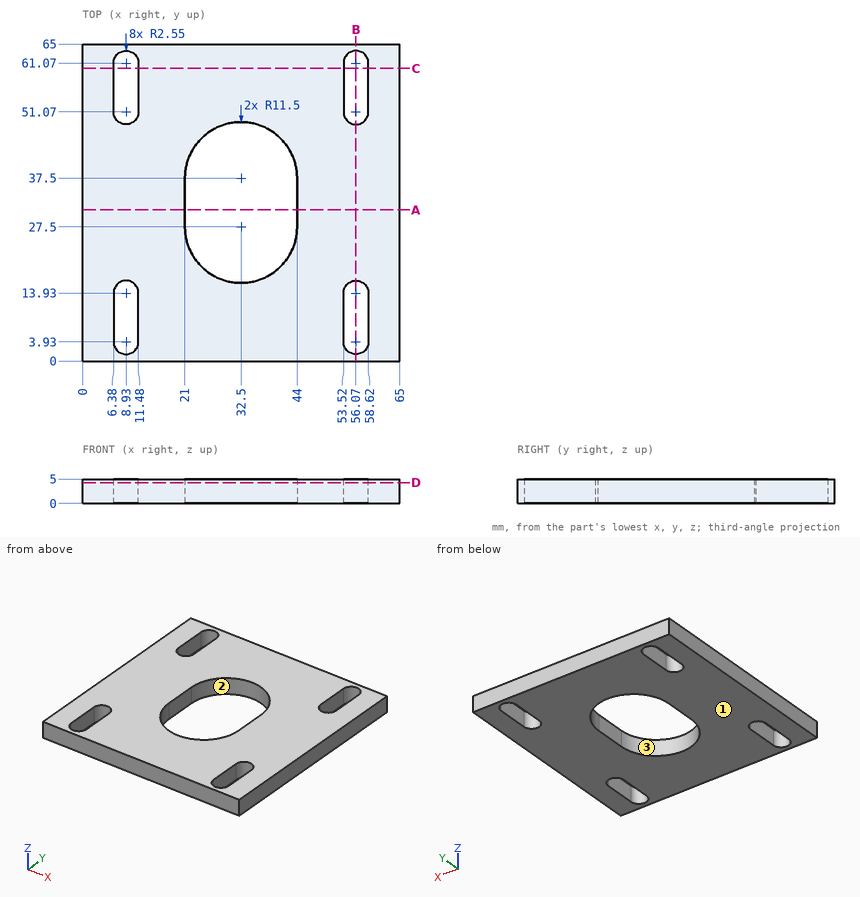
Here's the drawing with two shaded views (mm, measured from the low corner). I have some questions. Coordinates: 2 decimals unless noted, no trailing zeros. Order: outer loops, then holes, each group sorted by start corner. A loop starts at its lowest first (then second) coordinate and runs counter-clockwise, first axis right, second up. Notation, with made-up numbers: (84, 85) - (116, 85) arc R23 cw to (116, 107) - close; hole circle Ø3 at (61.5, -31). An arc over 180 degrees is marked (long way). Answer in a Markdown table with one row per item.
1. Suppose I cut it at D-D (z = 4.25). Please give me the cut outline in (x, y), and give its area (3 significant figures).
Reply:
| item | result |
|---|---|
| outline | (0, 0) - (65, 0) - (65, 65) - (0, 65) - close; hole (6.38, 3.93) arc R2.55 ccw to (11.48, 3.93) - (11.48, 13.93) arc R2.55 ccw to (6.38, 13.93) - close; hole (6.38, 51.07) arc R2.55 ccw to (11.48, 51.07) - (11.48, 61.07) arc R2.55 ccw to (6.38, 61.07) - close; hole (21, 27.5) arc R11.5 ccw to (44, 27.5) - (44, 37.5) arc R11.5 ccw to (21, 37.5) - close; hole (53.52, 3.93) arc R2.55 ccw to (58.62, 3.93) - (58.62, 13.93) arc R2.55 ccw to (53.52, 13.93) - close; hole (53.52, 51.07) arc R2.55 ccw to (58.62, 51.07) - (58.62, 61.07) arc R2.55 ccw to (53.52, 61.07) - close |
| area | 3,290 mm^2 |
2. Suppose I cut it at C-C (y = 60). Please give me the cut outline in (x, z), and give its area (3 significant figures).
Reply:
| item | result |
|---|---|
| outline | (0, 0) - (6.38, 0) - (6.38, 5) - (0, 5) - close; (11.48, 0) - (53.52, 0) - (53.52, 5) - (11.48, 5) - close; (58.62, 0) - (65, 0) - (65, 5) - (58.62, 5) - close |
| area | 274 mm^2 |
3. If I drill on line 1 along X through (y, z) = (52.5, 2.1); line 2 along X through (y, z) = (49.5, 1.65); line 3 along X through (y, z) = (34.5, 0.45), over which ranges is the centre line in solid material (lowest first)?
Reply:
| item | result |
|---|---|
| line 1 | x = 0 to 6.38, 11.48 to 53.52, 58.62 to 65 |
| line 2 | x = 0 to 6.92, 10.94 to 54.06, 58.08 to 65 |
| line 3 | x = 0 to 21, 44 to 65 |
4. If we mould it in two halves opening along Y, with no side actions, what happens to the marked faces 1, 2 and 3? For each: pulls with the +Y half, pulls with the -Y half, needs draft (parallel to the pull), parting line crosses it, or undercut.
Reply:
| item | result |
|---|---|
| face 1 | needs draft |
| face 2 | undercut |
| face 3 | undercut |
5. Suppose I cut it at B-B (x = 56.07). Please give me the cut outline in (y, z), and give its area (3 significant figures).
Reply:
| item | result |
|---|---|
| outline | (0, 0) - (1.38, 0) - (1.38, 5) - (0, 5) - close; (16.48, 0) - (48.52, 0) - (48.52, 5) - (16.48, 5) - close; (63.62, 0) - (65, 0) - (65, 5) - (63.62, 5) - close |
| area | 174 mm^2 |
6. Suppose I cut it at A-A (y = 31). Please give me the cut outline in (x, z), and give its area (3 significant figures).
Reply:
| item | result |
|---|---|
| outline | (0, 0) - (21, 0) - (21, 5) - (0, 5) - close; (44, 0) - (65, 0) - (65, 5) - (44, 5) - close |
| area | 210 mm^2 |
